Input: part model. Units: mm. Frame: model coordinates. Face numbers are marked on the shaded views. A direction names the side the tool comes from. Give positions to 0.01 mm unless a question says otherwise; leave off trailing zeros. Loops run counter-clockwise (first coordinate to the right, second up) from the corner with the lowest first, then second, coordinate; pieces in that order, holes last. Notation, with made-up numbers: M 62.5,-12.5 L 93.5,-12.5 A30 ccw 93.5,15.5 Z; hole C 19.25,16 d6. An arc over 180 degrees is marked long. Answer as a JSON object with one key per item and string values. Group by question number.
```python
from build123d import *

# Parameters (mm, degrees)
SKETCH2_R          = 2.5
CUT_EXTRUDE1_DEPTH = 29.026772914


with BuildPart() as part:
    # Sketch1 → Revolve1 (revolve)
    with BuildSketch(Plane.XY, mode=Mode.PRIVATE) as revolve1_sk:
        Polygon((0, 7), (0, 2.5), (8, 2.5), (8, 5), (3, 5), (3, 15.7), (4.5, 17.4), (4.5, 19.5), (-1.5, 19.5), (-1.5, 17.4), (0, 15.7), align=None)
        Polygon((-1, 2.5), (0, 2.5), (0, 7), (-1, 6), align=None)
    revolve(revolve1_sk.sketch.rotate(Axis((0, 0, 0), (1, 0, 0)), 90), axis=Axis((0, 0, 0), (1, 0, 0)))

    # Sketch2 → Cut-Extrude1 (cut, through all)
    with BuildSketch(Plane(origin=(3, 0, 0), x_dir=(0, 0, -1), z_dir=(1, 0, 0))):
        with Locations((0, 12)):
            Circle(SKETCH2_R)
        with Locations((8.485281374, 8.485281374)):
            Circle(SKETCH2_R)
        with Locations((12, 0)):
            Circle(SKETCH2_R)
        with Locations((8.485281374, -8.485281374)):
            Circle(SKETCH2_R)
        with Locations((0, -12)):
            Circle(SKETCH2_R)
        with Locations((-8.485281374, -8.485281374)):
            Circle(SKETCH2_R)
        with Locations((-12, 0)):
            Circle(SKETCH2_R)
        with Locations((-8.485281374, 8.485281374)):
            Circle(SKETCH2_R)
    extrude(amount=-CUT_EXTRUDE1_DEPTH, mode=Mode.SUBTRACT)


solid = part.part
```
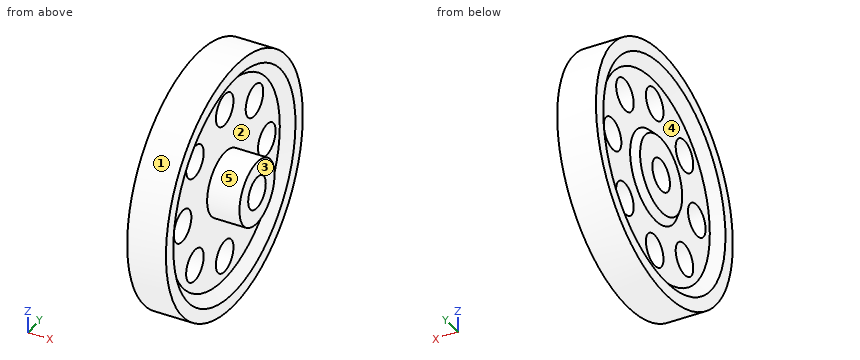
1. Section C-C (x = 7.25). Output: boundary loops of the cut face in (y, z).
2. Material intervals for L1, parallel to Y at x = 1.8, z = 0; L2, parallel to Y at x = 6.25, z = 0; L3, parallel to X at y = -10, z = -3.5, sorted ascending.
3. First-contact query: P1, Ø4, axis at y = -8.49, z = -8.49, coming from the -X side; P2, Ø6.5, axis at y = 0, z = -12, coming from the -X side; P3, Ø4, axis at x = 4.5, y = 13, coming from the -Z side; P4, Ø12, axis at y = -1, z = -7, coming from the -X side. Flat tips, straight axial feed; report the tip coordinate or a pass-through.
4. Section A-A (y = 0). Count the separate pieces of the cut face and the enclosed holes in it, then the cut area to 3 significant figures.
5. Reachability of the marked faces 4 and 5 from +Z, -Z, +X, -X, +Y, -Y: full face, straight path, thin tool, end or side. Return the list, or none.
6. Mould query, pull axis Y, two halves, no side actions, for the marked faces 1, 2 and 3. Classes: pulls with the +Y half, pulls with the -Y half, needs draft (parallel to the pull), parting line crosses it, or undercut.
Geometry results:
{
 "1": {"outline": "C 0,0 d10; hole C 0,0 d5"},
 "2": {"L1": "-19.5 to -14.5, -9.5 to -2.5, 2.5 to 9.5, 14.5 to 19.5", "L2": "-5 to -2.5, 2.5 to 5", "L3": "0 to 3"},
 "3": {"P1": "through", "P2": "x = 0", "P3": "z = -16.1", "P4": "x = -1"},
 "4": {"separate pieces": "4", "enclosed holes": "0", "area": "123 mm2"},
 "5": {"face 4": "-X", "face 5": "+X"},
 "6": {"face 1": "parting line crosses it", "face 2": "undercut", "face 3": "needs draft"}
}
